from build123d import *

# Parameters (mm, degrees)
F1_R     = 2.5
F2_DEPTH = 25
F6_DEPTH = 4


with BuildPart() as f2:
    # F1 (on Front) → F2 (new body)
    with BuildSketch(Plane.XZ):
        Circle(F1_R)
    extrude(amount=F2_DEPTH)

    # F3 (on Right) → F4 (revolve)
    with BuildSketch(Plane.YZ):
        with BuildLine():
            Line((0, 4.75), (0, 0))
            Line((0, 0), (3, 0))
            Line((3, 0), (3, 1.5))
            Line((3, 1.5), (3, 2.25))
            ThreePointArc((3, 2.25), (1.952562419, 4.0430749028), (0, 4.75))
        make_face()
    revolve(axis=Axis((0, 0, 0), (0, -1, 0)))

    # F5 (on face) → F6 (cut)
    with BuildSketch(Plane(origin=(0, 3, 0), x_dir=(-1, 0, 0), z_dir=(0, 1, 0))):
        Polygon((-1.5, 0.8660254038), (-1.5, -0.8660254038), (0, -1.7320508076), (1.5, -0.8660254038), (1.5, 0.8660254038), (0, 1.7320508076), align=None)
    extrude(amount=-F6_DEPTH, mode=Mode.SUBTRACT)


solid = f2.part
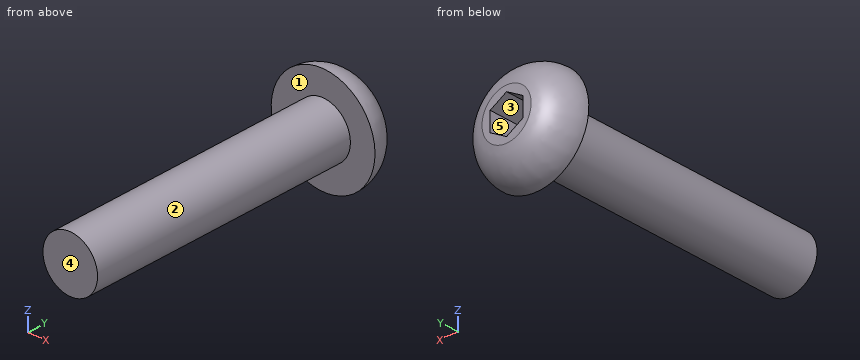
Geometry: final body of the model. Coordinates: model frame, mm. Face numbers are marked on the shaded views. A direction names the side the tool comes from. Give positions to 0.01 mm unless a question says otherwise; leave off trailing zeros. Write each loop counter-clockwise with the first axis right and the second up, starting at its lowest first coordinate (ties: lowest second). Pieces come first, ordered by that corner, then holes. Notation, with made-up numbers: (73.25, 81.5) -> (103.25, 81.5) arc R22 cw to (103.25, 99.5) -> close; hole circle Ø3 at (71, 30). An arc over 180 degrees is marked (long way). Answer as a JSON object with one key per item and string values.
1. Access query for the marked faces 4 and 5. Directions: +Z, -Z, +X, -X, +Y, -Y. A direction counts if a zero-diameter tool reaches every point of the face in a straight line with its end or side. Return the directions, or none.
Ans:
{"face 4": "+Z, -Z, +X, -X, -Y", "face 5": "+Y"}
2. Ray query, probe 1 along Z at (x, y) = (-2, -13.5); probe 2 along Y at (x, z) = (0.75, -0.25); probe 3 along X at (y, z) = (-11, -0.5). Return the intervals inside material, ascending. Write a range as from..to.
Ans:
{"probe 1": "z = -1.5..1.5", "probe 2": "y = -25..-1", "probe 3": "x = -2.45..2.45"}
3. Cut plane A-A on y = -14. Output: boundary loops of the cut face in (x, z).
Ans:
{"outline": "circle Ø5 at (0, 0)"}
4. Contact query for flat-ended pins moving along their axis: pin 1 (2 mm diameter, centred on y = -3.5, z = 0, fed in from -X); pin 2 (3 mm diameter, centred on x = -3, z = -2, fed in from -Y); pin 3 (2 mm diameter, centred on y = -11, z = -3, fed in from +X); pin 4 (2 mm diameter, centred on y = -13, z = -0.5, fed in from +X). Output: stop coordinate, or through.
Ans:
{"pin 1": "stops at x = -2.5", "pin 2": "stops at y = -25", "pin 3": "stops at x = 1.5", "pin 4": "stops at x = 2.5"}
5. Mould query, pull axis X, two halves, no side actions, for the marked faces 1, 2 and 3. Classes: pulls with the +X half, pulls with the -X half, needs draft (parallel to the pull), parting line crosses it, or undercut.
Ans:
{"face 1": "needs draft", "face 2": "parting line crosses it", "face 3": "undercut"}
